Part model, mm, in its own coordinate system. Coordinates: 2 decimals unless noted, no trailing zeros. Order: outer loops, then holes, each group sorted by start corner. A loop starts at its lowest first (then second) coordinate and runs counter-clockwise, first axis right, second up.
Autodesk Inventor part; units mm, degrees
ref_plane "YZ Plane" through (0, 0, 0) normal (1, 0, 0) x (0, 1, 0)
ref_plane "XZ Plane" through (0, 0, 0) normal (0, 1, 0) x (-1, 0, 0)
ref_plane "XY Plane" through (0, 0, 0) normal (0, 0, 1) x (1, 0, 0)
sketch "Sketch1" plane through (0, 0, 0) normal (0, 0, 1) x (1, 0, 0)
  circle A0 centre (0, 0) radius 7.5
  dimension "d0" = 15
extrude "Extrusion1" add sketch "Sketch1" along normal blind 35 draft -1
fillet "Fillet1" radius 2 2 edges at (-6.8891, 0, 35) (-7.5, 0, 0)
sketch "Sketch2" plane through (0, 0, 0) normal (0, 0, -1) x (-1, 0, 0)
  point P0 (0, 0)
sketch "Sketch3" plane through (0, 0, 0) normal (0, 0, -1) x (-1, 0, 0)
  circle A0 centre (0, 0) radius 4.9237
  line L0 (0, 0) -> (5.0385, 0)
  line L1 (5.0385, 0) -> (5.0385, 5)
  line L2 (5.0385, 5) -> (-5.7641, 5)
  line L3 (-5.7641, 5) -> (-5.7641, 0)
  circle A1 centre (0, 0) radius 6.9234
  line L4 (-5.7641, 0) -> (0, 0)
  dimension "d4" = 5
  dimension "d5" = 5
  dimension "d6" = 90
sketch "Sketch4" plane through (0, 0, 0) normal (0, 1, 0) x (-1, 0, 0)
  circle A0 centre (0, 30.571) radius 2.5
  point P0 (0, 0)
  dimension "d7" = 5
extrude "Extrusion2" cut sketch "Sketch4" against normal through all both and the other way through all
sketch "Sketch6" plane through (0, 0, 35) normal (0, 0, 1) x (1, 0, 0)
  arc A0 (-0.4232, 6.9104) -> (-0.4232, -6.9104) centre (0, 0) ccw
  line L0 (-4.7889, 5) -> (4.7889, 5)
  arc A1 (0.4232, -6.9104) -> (0.4232, 6.9104) centre (0, 0) ccw
  line L1 (-4.7889, 5) -> (-5.5424, 5)
  circle A2 centre (0, 0) radius 7.4645
  line L2 (4.7889, 5) -> (5.5429, 5)
  line L3 (-5.5424, -5) -> (5.5424, -5)
  arc A3 (-5.5424, 5) -> (-5.5424, -5) centre (0, 0) ccw
  arc A4 (5.5424, -5) -> (5.5429, 5) centre (-0.0007, 0.0003) ccw
  point P0 (0, 0)
  dimension "d14" = 5
  dimension "d15" = 5
extrude "Extrusion4" cut sketch "Sketch6" against normal blind 12 contours L0 A1 L3 A0 | A0 L3 A2 L1 | L2 A2 L3 A1
chamfer "Chamfer1" distance 2 angle 45 2 edges at (6.5634, -2.7038, 23) (-7.0985, 0, 23)
sketch "Sketch7" plane through (0, 0, 0) normal (0, 1, 0) x (-1, 0, 0)
  point P0 (0, 0)
properties part number "bicep"
Q1. Wall check: line 1 along Z through (x, y) = (-3.25, -3.25); line 2 along Z through (x, y) = (0, 6.25); line 3 along Z through (x, y) = (0, -6.35). Give the ranges that are in metal, low to high.
Results list:
line 1: z = 0 to 23
line 2: z = 0.16 to 28.07, 33.07 to 34.5
line 3: z = 0.21 to 28.07, 33.07 to 34.4
Q2. Cut at A-A on x = 0. Count the separate pieces of the cut face and the enclosed holes in it, and give its area (3 significant figures).
Results list:
separate pieces: 3
enclosed holes: 0
area: 361 mm2
Q3. Pin check, flat tips, straight feed: pin 1 Ø3 at (x, z) = (0, 30.571) entering from +Y; pin 2 Ø5 at (x, z) = (-0.5, 18) entering from +Y; pin 3 Ø3 at (x, z) = (0, 25.5) entering from +Y; pin 4 Ø6 at (x, z) = (5.5, 31) entering from +Y. Stop position of each tip, or through.
Results list:
pin 1: passes through
pin 2: stops at y = 7.23
pin 3: stops at y = 7.08
pin 4: stops at y = 6.5
Q4. Cut at B-B on z = 6.5. Write the cut outline in (x, y).
Results list:
outline: circle Ø14.77 at (0, 0)
Q5. Mould opens along X. For faces 1 (the face through (6.923, -2.18, 13.873)), 2 (the face through (1.984, 5.796, 29.05)), 3 (the face through (0, 0, 23)), 4 (the face through (1.984, -5.991, 29.05)) say: pulls with the +X half, pulls with the -X half, needs draft (parallel to the pull), parting line crosses it, or undercut.
Results list:
face 1: parting line crosses it
face 2: undercut
face 3: needs draft
face 4: undercut
